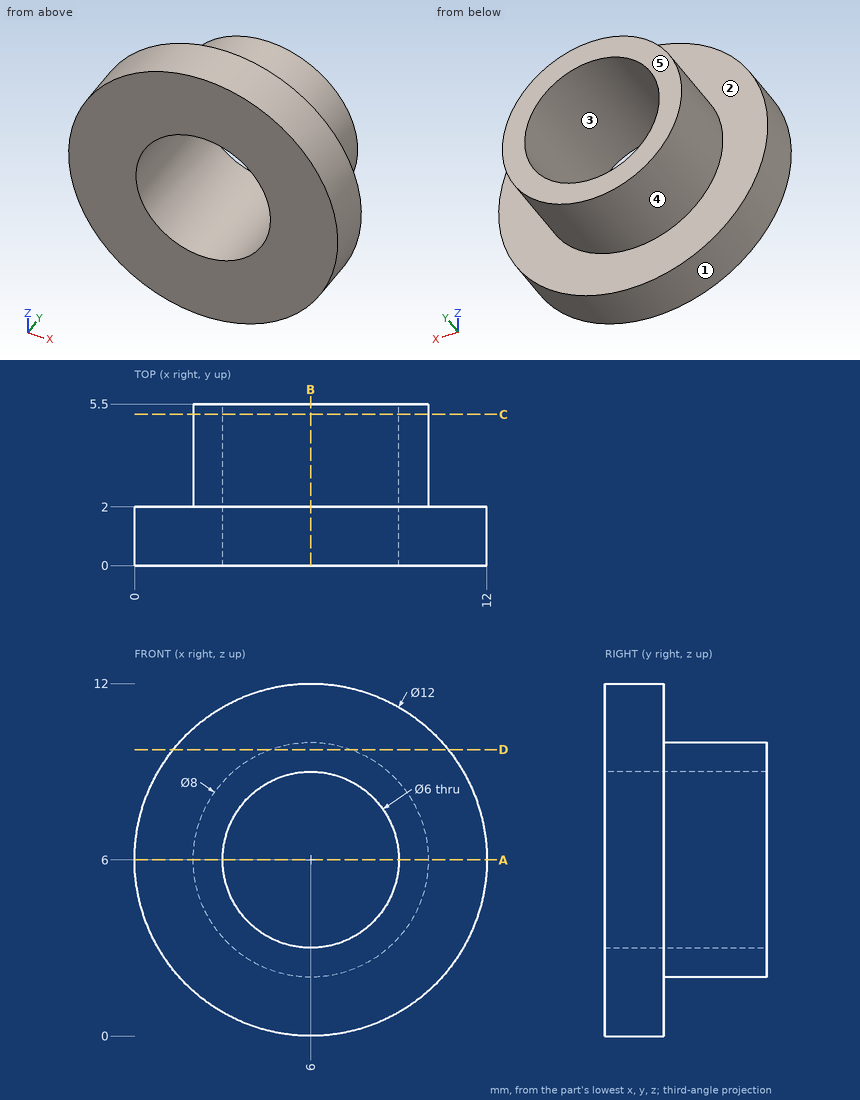
Job drawing, mm, ordinate dimensions from the low corner. One solid piece. A direction names the side the tool comes from. Round coordinates to 2 decimals unless told otherwise and drop trailing zeros. Order: outer loops, then holes, each group sorted by start corner. A loop starts at its lowest first (then second) coordinate and runs counter-clockwise, first axis right, second up. Notation, with made-up numbers: (20, 29) - (58, 29) arc R9 ccw to (58, 43) - close; hole circle Ø4 at (78.5, 35.5). An arc over 180 degrees is marked (long way). Use CSV: the item, a comma, the result in double quotes. Start each with the question number.
1) Saw through at D-D (z = 9.75). List the corners of the cut face in (x, y).
2) Saw through at B-B (x = 6). List the corners of the cut face in (y, z).
3) Two-plate mould, pull along Z, no slides. Class the marked faces 3, 4 and 5: pulls with the +Z half, pulls with the -Z half, needs draft (parallel to the pull), parting line crosses it, or undercut.
4) Pin check, flat tips, straight feed: pin 1 Ø2 at (y, z) = (4, 6.5) entering from +X; pin 2 Ø1.5 at (y, z) = (3.5, 8) entering from -X. Stop position of each tip, or through.
5) Saw through at C-C (y = 5.15). List the corners of the cut face in (x, z).
6) Tool access for the marked faces 1 and 2: list every direction of +Z, -Z, +X, -X, +Y, -Y with a clear straight run to the whole face (end or side of a thin tool).
7) Wall check: L1, parallel to X at y = 3.35, z = 6; L2, parallel to X at y = 1.5, z = 6; L3, parallel to Y at x = 9, z = 9. Give the ranges that are in metal, low to high. Write a range as [from, to].
8) Saw through at A-A (z = 6). List the corners of the cut face in (x, y).
Values follow:
1,outline,"(1.32, 0) - (10.68, 0) - (10.68, 2) - (7.39, 2) - (7.39, 5.5) - (4.61, 5.5) - (4.61, 2) - (1.32, 2) - close"
2,outline,"(0, 0) - (2, 0) - (2, 2) - (5.5, 2) - (5.5, 3) - (0, 3) - close; (0, 9) - (5.5, 9) - (5.5, 10) - (2, 10) - (2, 12) - (0, 12) - close"
3,face 3,"undercut"
3,face 4,"parting line crosses it"
3,face 5,"needs draft"
4,pin 1,"stops at x = 10"
4,pin 2,"stops at x = 2.2"
5,outline,"circle Ø8 at (6, 6); hole circle Ø6 at (6, 6)"
6,face 1,"+Y, -Y"
6,face 2,"+Y"
7,L1,"x = [2, 3], [9, 10]"
7,L2,"x = [0, 3], [9, 12]"
7,L3,"y = [0, 2]"
8,outline,"(0, 0) - (3, 0) - (3, 5.5) - (2, 5.5) - (2, 2) - (0, 2) - close; (9, 0) - (12, 0) - (12, 2) - (10, 2) - (10, 5.5) - (9, 5.5) - close"
